```python
from build123d import *

# Parameters (mm, degrees)
SKETCH1_R           = 6.875
BOSS_EXTRUDE1_DEPTH = 20
SKETCH2_W           = 2.41756572
SKETCH2_H           = 10
BOSS_EXTRUDE2_DEPTH = 30
SKETCH3_R           = 7
BOSS_EXTRUDE3_DEPTH = 25


with BuildPart() as part:
    # Sketch1 → Boss-Extrude1 (new body)
    with BuildSketch(Plane(origin=(0, 0, 0), x_dir=(1, 0, 0), z_dir=(0, 1, 0))):
        Circle(SKETCH1_R)
    extrude(amount=BOSS_EXTRUDE1_DEPTH)

    # Sketch2 → Boss-Extrude2 (add)
    with BuildSketch(Plane(origin=(0, 0, 0), x_dir=(0, 0, -1), z_dir=(1, 0, 0))):
        with Locations((0, 20)):
            Rectangle(SKETCH2_W, SKETCH2_H)
    extrude(amount=BOSS_EXTRUDE2_DEPTH)

    # Sketch3 → Boss-Extrude3 (add)
    with BuildSketch(Plane.XY):
        with Locations((30, 20)):
            Circle(SKETCH3_R)
    extrude(amount=BOSS_EXTRUDE3_DEPTH)


solid = part.part
```
For this review, take the finished solid that the model builds, in its own axes (mm). A direction names the side the tool comes from. Coordinates: 2 decimals unless noted, no trailing zeros. Write each loop counter-clockwise with the first axis right and the second up, starting at its lowest first coordinate (ties: lowest second). Pieces come first, ordered by that corner, then holes.
(1) Add section A-A on z = 17.5. Give the boundary of the cut face in (x, y).
(2) Add section D-D on x = 30.5. Give the boundary of the cut face in (y, z), then the cut area to 3 significant figures.
(3) Wall thickness on probe 1 along X at (y, z) = (19.5, 3.5); probe 2 along Z at (x, y) = (31, 25.5); probe 3 along X at (y, z) = (19.25, 10.5): over which ranges is each line inside the solid? List them lowest first.
(4) The part is to be moulded in two halves that separate along X. For faces 1 (the face through (0, 0, 0)), 2 (the face through (0, 23, 0)), 3 (the face through (30, 20, -1)), 4 (the face through (18, 15, 0)), say which applies: +X half, -X half, draft (parallel to the pull), parting line (faces both ways), or undercut.
(5) For pin 1 Ø5 at (x, y) = (6, 17.5) entering from -Z; pin 2 Ø3.5 at (x, y) = (29.5, 20.5) entering from -Z; pin 3 Ø2.5 at (x, z) = (23, 0.5) entering from -Y; pin 4 Ø6 at (y, z) = (5, 12) entering from -X, all flat-tipped, find the tip position at first contact; note any pin that passes through.
(6) Add section B-B on y = 4.5. Give the boundary of the cut face in (x, z) (3 decimals), then the cut area to 3 significant figures.
(7) Tool access review of faces 5 (the face through (33.23, 13.79, 12.32)), 6 (the face through (30, 20, 25)): name each direction out of +Z, -Z, +X, -X, +Y, -Y from which nothing blocks a thin tool from reaching the whole face with its end or side.
(8) Add section C-C on z = 3.5. Give the boundary of the cut face in (x, y).
Answer sheet:
1. outline: circle Ø14 at (30, 20)
2. outline: (13.02, 0) - (26.98, 0) - (26.98, 25) - (13.02, 25) - close
2. area: 349 mm2
3. probe 1: x = -5.92 to 5.92, 23.02 to 36.98
3. probe 2: z = 0 to 25
3. probe 3: x = 23.04 to 36.96
4. face 1: draft
4. face 2: -X half
4. face 3: +X half
4. face 4: undercut
5. pin 1: stops at z = -5.92
5. pin 2: stops at z = -1.21
5. pin 3: stops at y = 15
5. pin 4: passes through
6. outline: circle Ø13.75 at (0, 0)
6. area: 148 mm2
7. face 5: +Z
7. face 6: +Z, +X, -X, +Y, -Y
8. outline: (-5.92, 0) - (5.92, 0) - (5.92, 20) - (-5.92, 20) - close; circle Ø14 at (30, 20)
